Design review of the part built by this model. Coordinates are the model's own, in mm. A direction names the side the tool comes from. Round coordinates to 2 decimals unless told otherwise and drop trailing zeros. One line per question, with ' | ' between items. Start each with the question number.
Item 1: Machinability: for faces 3 (the face through (50, 44, -56)), 4 (the face through (83.43, 38.93, -67.12)), which of the approach directions +Z, -Z, +X, -X, +Y, -Y give a long, thin tool a straight path to every point of the face, cutting with its end or side? Answer none if there is none.
Item 2: For L1, parallel to Y at x = 68, z = -79, list the stretches that pass through material, from the lowest coordinate up.
Item 3: Insertion check: pin 1 Ø5 at (y, z) = (38, -14) entering from -X. The pin has a flat end and moves straight along its axis. Give the tip position at first contact, or say it passes through.
Item 4: Draft analysis for pull direction X (two halves, no side actions). For faces 1 (the face through (86, 44, -38)), 2 (the face through (96.721, 38.93, -59.473)), state which applies: released by +X, released by -X, zero draft, split by the parting line, or undercut.
```python
from build123d import *

# Parameters (mm, degrees)
SKETCH1_W           = 127
SKETCH1_H           = 84.582
BOSS_EXTRUDE1_DEPTH = 34
SKETCH4_R           = 3.5
BOSS_EXTRUDE2_DEPTH = 10


with BuildPart() as part:
    # Sketch1 → Boss-Extrude1 (new body)
    with BuildSketch(Plane(origin=(0, 0, 0), x_dir=(1, 0, 0), z_dir=(0, 1, 0))):
        with Locations((63.5, 42.291)):
            Rectangle(SKETCH1_W, SKETCH1_H)
    extrude(amount=BOSS_EXTRUDE1_DEPTH)

    # Sketch4 → Boss-Extrude2 (add)
    with BuildSketch(Plane(origin=(0, 34, 0), x_dir=(1, 0, 0), z_dir=(0, 1, 0))):
        with Locations(Location((104.38, 11.24, 0), (0, 0, 90))):
            Circle(SKETCH4_R)
        with Locations(Location((95.38, 11.24, 0), (0, 0, 90))):
            Circle(SKETCH4_R)
        with Locations(Location((86.38, 11.24, 0), (0, 0, 90))):
            Circle(SKETCH4_R)
        with Locations(Location((77.38, 11.24, 0), (0, 0, 90))):
            Circle(SKETCH4_R)
        with Locations(Location((68.38, 11.24, 0), (0, 0, 90))):
            Circle(SKETCH4_R)
        with Locations(Location((59.38, 11.24, 0), (0, 0, 90))):
            Circle(SKETCH4_R)
        with Locations(Location((50.38, 11.24, 0), (0, 0, 90))):
            Circle(SKETCH4_R)
        with Locations(Location((41.38, 11.24, 0), (0, 0, 90))):
            Circle(SKETCH4_R)
        with Locations(Location((32.38, 11.24, 0), (0, 0, 90))):
            Circle(SKETCH4_R)
        with Locations(Location((23.38, 11.24, 0), (0, 0, 90))):
            Circle(SKETCH4_R)
        with Locations(Location((14.38, 11.24, 0), (0, 0, 90))):
            Circle(SKETCH4_R)
        with Locations(Location((113.38, 20.24, 0), (0, 0, 90))):
            Circle(SKETCH4_R)
        with Locations(Location((104.38, 20.24, 0), (0, 0, 90))):
            Circle(SKETCH4_R)
        with Locations(Location((95.38, 20.24, 0), (0, 0, 90))):
            Circle(SKETCH4_R)
        with Locations(Location((86.38, 20.24, 0), (0, 0, 90))):
            Circle(SKETCH4_R)
        with Locations(Location((77.38, 20.24, 0), (0, 0, 90))):
            Circle(SKETCH4_R)
        with Locations(Location((68.38, 20.24, 0), (0, 0, 90))):
            Circle(SKETCH4_R)
        with Locations(Location((59.38, 20.24, 0), (0, 0, 90))):
            Circle(SKETCH4_R)
        with Locations(Location((50.38, 20.24, 0), (0, 0, 90))):
            Circle(SKETCH4_R)
        with Locations(Location((41.38, 20.24, 0), (0, 0, 90))):
            Circle(SKETCH4_R)
        with Locations(Location((32.38, 20.24, 0), (0, 0, 90))):
            Circle(SKETCH4_R)
        with Locations(Location((23.38, 20.24, 0), (0, 0, 90))):
            Circle(SKETCH4_R)
        with Locations(Location((14.38, 20.24, 0), (0, 0, 90))):
            Circle(SKETCH4_R)
        with Locations(Location((113.38, 29.24, 0), (0, 0, 90))):
            Circle(SKETCH4_R)
        with Locations(Location((104.38, 29.24, 0), (0, 0, 90))):
            Circle(SKETCH4_R)
        with Locations(Location((95.38, 29.24, 0), (0, 0, 90))):
            Circle(SKETCH4_R)
        with Locations(Location((113.38, 11.24, 0), (0, 0, 90))):
            Circle(SKETCH4_R)
        with Locations(Location((86.38, 29.24, 0), (0, 0, 90))):
            Circle(SKETCH4_R)
        with Locations(Location((77.38, 29.24, 0), (0, 0, 90))):
            Circle(SKETCH4_R)
        with Locations(Location((68.38, 29.24, 0), (0, 0, 90))):
            Circle(SKETCH4_R)
        with Locations(Location((59.38, 29.24, 0), (0, 0, 90))):
            Circle(SKETCH4_R)
        with Locations(Location((50.38, 29.24, 0), (0, 0, 90))):
            Circle(SKETCH4_R)
        with Locations(Location((41.38, 29.24, 0), (0, 0, 90))):
            Circle(SKETCH4_R)
        with Locations(Location((32.38, 29.24, 0), (0, 0, 90))):
            Circle(SKETCH4_R)
        with Locations(Location((23.38, 29.24, 0), (0, 0, 90))):
            Circle(SKETCH4_R)
        with Locations(Location((14.38, 29.24, 0), (0, 0, 90))):
            Circle(SKETCH4_R)
        with Locations(Location((113.38, 38.24, 0), (0, 0, 90))):
            Circle(SKETCH4_R)
        with Locations(Location((104.38, 38.24, 0), (0, 0, 90))):
            Circle(SKETCH4_R)
        with Locations(Location((95.38, 38.24, 0), (0, 0, 90))):
            Circle(SKETCH4_R)
        with Locations(Location((86.38, 38.24, 0), (0, 0, 90))):
            Circle(SKETCH4_R)
        with Locations(Location((77.38, 38.24, 0), (0, 0, 90))):
            Circle(SKETCH4_R)
        with Locations(Location((68.38, 38.24, 0), (0, 0, 90))):
            Circle(SKETCH4_R)
        with Locations(Location((59.38, 38.24, 0), (0, 0, 90))):
            Circle(SKETCH4_R)
        with Locations(Location((50.38, 38.24, 0), (0, 0, 90))):
            Circle(SKETCH4_R)
        with Locations(Location((41.38, 38.24, 0), (0, 0, 90))):
            Circle(SKETCH4_R)
        with Locations(Location((32.38, 38.24, 0), (0, 0, 90))):
            Circle(SKETCH4_R)
        with Locations(Location((23.38, 38.24, 0), (0, 0, 90))):
            Circle(SKETCH4_R)
        with Locations(Location((14.38, 38.24, 0), (0, 0, 90))):
            Circle(SKETCH4_R)
        with Locations(Location((113.38, 47.24, 0), (0, 0, 90))):
            Circle(SKETCH4_R)
        with Locations(Location((104.38, 47.24, 0), (0, 0, 90))):
            Circle(SKETCH4_R)
        with Locations(Location((95.38, 47.24, 0), (0, 0, 90))):
            Circle(SKETCH4_R)
        with Locations(Location((86.38, 47.24, 0), (0, 0, 90))):
            Circle(SKETCH4_R)
        with Locations(Location((77.38, 47.24, 0), (0, 0, 90))):
            Circle(SKETCH4_R)
        with Locations(Location((68.38, 47.24, 0), (0, 0, 90))):
            Circle(SKETCH4_R)
        with Locations(Location((59.38, 47.24, 0), (0, 0, 90))):
            Circle(SKETCH4_R)
        with Locations(Location((50.38, 47.24, 0), (0, 0, 90))):
            Circle(SKETCH4_R)
        with Locations(Location((41.38, 47.24, 0), (0, 0, 90))):
            Circle(SKETCH4_R)
        with Locations(Location((32.38, 47.24, 0), (0, 0, 90))):
            Circle(SKETCH4_R)
        with Locations(Location((23.38, 47.24, 0), (0, 0, 90))):
            Circle(SKETCH4_R)
        with Locations(Location((14.38, 47.24, 0), (0, 0, 90))):
            Circle(SKETCH4_R)
        with Locations(Location((113.38, 56.24, 0), (0, 0, 90))):
            Circle(SKETCH4_R)
        with Locations(Location((104.38, 56.24, 0), (0, 0, 90))):
            Circle(SKETCH4_R)
        with Locations(Location((95.38, 56.24, 0), (0, 0, 90))):
            Circle(SKETCH4_R)
        with Locations(Location((86.38, 56.24, 0), (0, 0, 90))):
            Circle(SKETCH4_R)
        with Locations(Location((77.38, 56.24, 0), (0, 0, 90))):
            Circle(SKETCH4_R)
        with Locations(Location((68.38, 56.24, 0), (0, 0, 90))):
            Circle(SKETCH4_R)
        with Locations(Location((59.38, 56.24, 0), (0, 0, 90))):
            Circle(SKETCH4_R)
        with Locations(Location((50.38, 56.24, 0), (0, 0, 90))):
            Circle(SKETCH4_R)
        with Locations(Location((41.38, 56.24, 0), (0, 0, 90))):
            Circle(SKETCH4_R)
        with Locations(Location((32.38, 56.24, 0), (0, 0, 90))):
            Circle(SKETCH4_R)
        with Locations(Location((23.38, 56.24, 0), (0, 0, 90))):
            Circle(SKETCH4_R)
        with Locations(Location((14.38, 56.24, 0), (0, 0, 90))):
            Circle(SKETCH4_R)
        with Locations(Location((113.38, 65.24, 0), (0, 0, 90))):
            Circle(SKETCH4_R)
        with Locations(Location((104.38, 65.24, 0), (0, 0, 90))):
            Circle(SKETCH4_R)
        with Locations(Location((95.38, 65.24, 0), (0, 0, 90))):
            Circle(SKETCH4_R)
        with Locations(Location((86.38, 65.24, 0), (0, 0, 90))):
            Circle(SKETCH4_R)
        with Locations(Location((77.38, 65.24, 0), (0, 0, 90))):
            Circle(SKETCH4_R)
        with Locations(Location((68.38, 65.24, 0), (0, 0, 90))):
            Circle(SKETCH4_R)
        with Locations(Location((59.38, 65.24, 0), (0, 0, 90))):
            Circle(SKETCH4_R)
        with Locations(Location((50.38, 65.24, 0), (0, 0, 90))):
            Circle(SKETCH4_R)
        with Locations(Location((41.38, 65.24, 0), (0, 0, 90))):
            Circle(SKETCH4_R)
        with Locations(Location((32.38, 65.24, 0), (0, 0, 90))):
            Circle(SKETCH4_R)
        with Locations(Location((23.38, 65.24, 0), (0, 0, 90))):
            Circle(SKETCH4_R)
        with Locations(Location((14.38, 65.24, 0), (0, 0, 90))):
            Circle(SKETCH4_R)
        with Locations(Location((113.38, 74.24, 0), (0, 0, 90))):
            Circle(SKETCH4_R)
        with Locations(Location((104.38, 74.24, 0), (0, 0, 90))):
            Circle(SKETCH4_R)
        with Locations(Location((95.38, 74.24, 0), (0, 0, 90))):
            Circle(SKETCH4_R)
        with Locations(Location((86.38, 74.24, 0), (0, 0, 90))):
            Circle(SKETCH4_R)
        with Locations(Location((77.38, 74.24, 0), (0, 0, 90))):
            Circle(SKETCH4_R)
        with Locations(Location((68.38, 74.24, 0), (0, 0, 90))):
            Circle(SKETCH4_R)
        with Locations(Location((59.38, 74.24, 0), (0, 0, 90))):
            Circle(SKETCH4_R)
        with Locations(Location((50.38, 74.24, 0), (0, 0, 90))):
            Circle(SKETCH4_R)
        with Locations(Location((41.38, 74.24, 0), (0, 0, 90))):
            Circle(SKETCH4_R)
        with Locations(Location((32.38, 74.24, 0), (0, 0, 90))):
            Circle(SKETCH4_R)
        with Locations(Location((23.38, 74.24, 0), (0, 0, 90))):
            Circle(SKETCH4_R)
        with Locations(Location((14.38, 74.24, 0), (0, 0, 90))):
            Circle(SKETCH4_R)
    extrude(amount=BOSS_EXTRUDE2_DEPTH)


solid = part.part
```
Computed values:
1) face 3: +Z, -Z, +X, -X, +Y | face 4: +Y
2) L1: y = 0 to 34
3) pin 1: stops at x = 10.89
4) face 1: zero draft | face 2: undercut
